from build123d import *

# Parameters (mm, degrees)
SALIENTE_EXTRUIR1_DEPTH = 4.5
CROQUIS4_R              = 17
CROQUIS4_R_2            = 2
CORTAR_EXTRUIR3_DEPTH   = 599.217436148
CHAFL_N1_SIZE           = 0.5
CROQUIS5_R              = 8
CROQUIS5_R_2            = 3
CORTAR_EXTRUIR4_DEPTH   = 599.217436148
CHAFL_N2_SIZE           = 0.5
CROQUIS3_R              = 3
CORTAR_EXTRUIR2_DEPTH   = 599.217436148
CHAFL_N3_SIZE           = 0.5
CROQUIS2_R              = 2
CORTAR_EXTRUIR1_DEPTH   = 599.217436148
CHAFL_N4_SIZE           = 0.5


with BuildPart() as part:
    # Croquis1 → Saliente-Extruir1 (new, symmetric)
    with BuildSketch(Plane(origin=(0, 0, 0), x_dir=(0, 0, -1), z_dir=(1, 0, 0))):
        Polygon((-294.796624044, -440.459461787), (-174.796624044, -290.459461787), (-174.796624044, -150.459461787), (-114.796624044, -150.459461787), (-114.796624044, -350.459461787), (-174.796624044, -440.459461787), (-174.796624044, -520.459461787), (-294.796624044, -520.459461787), align=None)
    extrude(amount=SALIENTE_EXTRUIR1_DEPTH, both=True)

    # Croquis4 → Cortar-Extruir3 (cut, through all)
    with BuildSketch(Plane(origin=(4.5, 0, 0), x_dir=(0, 0, -1), z_dir=(1, 0, 0))):
        with Locations((-143.796624044, -224.459461787)):
            Circle(CROQUIS4_R)
        with Locations((-158.645866449, -209.610219382)):
            Circle(CROQUIS4_R_2)
        with Locations((-128.947381639, -209.610219382)):
            Circle(CROQUIS4_R_2)
        with Locations((-128.947381639, -239.308704192)):
            Circle(CROQUIS4_R_2)
        with Locations((-158.645866449, -239.308704192)):
            Circle(CROQUIS4_R_2)
    extrude(amount=-CORTAR_EXTRUIR3_DEPTH, mode=Mode.SUBTRACT)

    # Chaflán1
    chafl_n1_edges = [part.edges().sort_by_distance(p)[0] for p in [
        (-4.5, -209.610219382, 160.645866449),
        (-4.5, -224.459461787, 160.796624044),
        (4.5, -224.459461787, 160.796624044),
        (-4.5, -209.610219382, 130.947381639),
        (-4.5, -239.308704192, 130.947381639),
        (-4.5, -239.308704192, 160.645866449),
    ]]
    chamfer(chafl_n1_edges, length=CHAFL_N1_SIZE)

    # Croquis5 → Cortar-Extruir4 (cut, through all)
    with BuildSketch(Plane(origin=(4.5, 0, 0), x_dir=(0, 0, -1), z_dir=(1, 0, 0))):
        with Locations((-144.796624044, -170.459461787)):
            Circle(CROQUIS5_R)
        with Locations((-144.796624044, -278.459461787)):
            Circle(CROQUIS5_R)
        with Locations((-124.796624044, -170.459461787)):
            Circle(CROQUIS5_R_2)
        with Locations((-164.796624044, -170.459461787)):
            Circle(CROQUIS5_R_2)
        with Locations((-164.796624044, -278.459461787)):
            Circle(CROQUIS5_R_2)
        with Locations((-124.796624044, -278.459461787)):
            Circle(CROQUIS5_R_2)
    extrude(amount=-CORTAR_EXTRUIR4_DEPTH, mode=Mode.SUBTRACT)

    # Chaflán2
    chafl_n2_edges = [part.edges().sort_by_distance(p)[0] for p in [
        (-4.5, -170.459461787, 152.796624044),
        (4.5, -170.459461787, 152.796624044),
        (-4.5, -278.459461787, 152.796624044),
        (4.5, -278.459461787, 152.796624044),
        (-4.5, -170.459461787, 127.796624044),
        (-4.5, -170.459461787, 167.796624044),
        (-4.5, -278.459461787, 167.796624044),
        (-4.5, -278.459461787, 127.796624044),
    ]]
    chamfer(chafl_n2_edges, length=CHAFL_N2_SIZE)

    # Croquis3 → Cortar-Extruir2 (cut, through all)
    with BuildSketch(Plane(origin=(4.5, 0, 0), x_dir=(0, 0, -1), z_dir=(1, 0, 0))):
        with Locations((-289.796624044, -473.459461787)):
            Circle(CROQUIS3_R)
        with Locations((-289.796624044, -513.459461787)):
            Circle(CROQUIS3_R)
        with Locations((-249.796624044, -473.459461787)):
            Circle(CROQUIS3_R)
        with Locations((-249.796624044, -513.459461787)):
            Circle(CROQUIS3_R)
        with Locations(Location((-219.796624044, -513.459461787, 0), (0, 0, 180))):
            Circle(CROQUIS3_R)
        with Locations(Location((-219.796624044, -473.459461787, 0), (0, 0, 180))):
            Circle(CROQUIS3_R)
        with Locations(Location((-179.796624044, -513.459461787, 0), (0, 0, 180))):
            Circle(CROQUIS3_R)
        with Locations(Location((-179.796624044, -473.459461787, 0), (0, 0, 180))):
            Circle(CROQUIS3_R)
    extrude(amount=-CORTAR_EXTRUIR2_DEPTH, mode=Mode.SUBTRACT)

    # Chaflán3
    chafl_n3_edges = [part.edges().sort_by_distance(p)[0] for p in [
        (-4.5, -473.459461787, 292.796624044),
        (-4.5, -513.459461787, 292.796624044),
        (-4.5, -473.459461787, 252.796624044),
        (-4.5, -513.459461787, 252.796624044),
        (-4.5, -513.459461787, 216.796624044),
        (-4.5, -473.459461787, 216.796624044),
        (-4.5, -513.459461787, 176.796624044),
        (-4.5, -473.459461787, 176.796624044),
    ]]
    chamfer(chafl_n3_edges, length=CHAFL_N3_SIZE)

    # Croquis2 → Cortar-Extruir1 (cut, through all)
    with BuildSketch(Plane(origin=(4.5, 0, 0), x_dir=(0, 0, -1), z_dir=(1, 0, 0))):
        with Locations((-234.796624044, -460.459461787)):
            Circle(CROQUIS2_R)
        with Locations((-269.796624044, -460.459461787)):
            Circle(CROQUIS2_R)
        with Locations((-199.796624044, -460.459461787)):
            Circle(CROQUIS2_R)
    extrude(amount=-CORTAR_EXTRUIR1_DEPTH, mode=Mode.SUBTRACT)

    # Chaflán4
    chafl_n4_edges = [part.edges().sort_by_distance(p)[0] for p in [
        (-4.5, -460.459461787, 236.796624044),
        (-4.5, -460.459461787, 271.796624044),
        (-4.5, -460.459461787, 201.796624044),
    ]]
    chamfer(chafl_n4_edges, length=CHAFL_N4_SIZE)


solid = part.part
The listing builds one solid part. Answer for the finished solid, in the listing's coordinates (mm). Give positions to 0.01 mm unless a question says otherwise; leave off trailing zeros. Write each loop counter-clockwise with the first axis right and the second up, starting at its lowest first coordinate (ties: lowest second). Pieces come first, ordered by that corner, then holes. Notation, with made-up numbers: (81.5, 1.5) -> (130.5, 1.5) arc R25 cw to (130.5, 30.5) -> close; hole circle Ø4 at (7, -9). An arc over 180 degrees is marked (long way). One line per question, with ' | ' between items. Start each with the question number.
1. Section B-B (y = -249) is taken. Determine the outline of the cut face in (x, z).
2. For a pull along Y with two mould halves and no side action, classify faces 1 (the cylindrical face through (0.06, -223.71, 160.78)), 2 (the flat face through (0.063, -366.509, 235.637)), 3 (the cylindrical face through (0.06, -170.11, 152.79)), 4 (the flat face through (0, -221, 174.797)) as pulls with the +Y half, pulls with the -Y half, needs draft (parallel to the pull), parting line crosses it, or undercut.
3. Given pin 1 Ø5.5 at (y, z) = (-513.46, 289.8) entering from +X; pin 2 Ø5 at (y, z) = (-209.61, 128.95) entering from +X; pin 3 Ø4.5 at (y, z) = (-239.31, 128.95) entering from -X; pin 4 Ø1 at (x, z) = (-3, 158.5) entering from -Y, each flat-ended and moving along its own axis, determine where each tip first touches the part or whether it passes through.
4. Section A-A (x = -1) is taken. State how many separate pieces and enclosed holes the cut face has, plus the area to 3 significant figures.
5. Section D-D (z = 208) is taken. Determine the outline of the cut face in (x, y).
6. Find the intervals of material crossed by probe 1 along Y at (x, z) = (0.25, 138.5); probe 2 along Y at (x, z) = (-1.75, 158); probe 3 along Y at (x, z) = (-2.25, 163), in increasing order.
Response values:
1) outline: (-4.5, 114.8) -> (4.5, 114.8) -> (4.5, 174.8) -> (-4.5, 174.8) -> close
2) face 1: undercut | face 2: pulls with the +Y half | face 3: undercut | face 4: needs draft
3) pin 1: through | pin 2: x = 4.5 | pin 3: x = -4.25 | pin 4: y = -416.76
4) separate pieces: 1 | enclosed holes: 22 | area: 31,600 mm2
5) outline: (-4.5, -520.46) -> (4.5, -520.46) -> (4.5, -331.96) -> (-4.5, -331.96) -> close
6) probe 1: -386.01 to -283.39, -273.52 to -240.61, -208.31 to -175.39, -165.52 to -150.46 | probe 2: -415.26 to -241.2, -237.42 to -233.8, -215.12 to -211.5, -207.72 to -150.46 | probe 3: -422.76 to -280.86, -276.06 to -172.86, -168.06 to -150.46
